from build123d import *

# Parameters (mm, degrees)
EXTRUDE1_DEPTH      = 228.73
CUT_EXTRUDE1_DEPTH  = 95
EXTRUDE2_DEPTH      = 50
EXTRUDE2_DEPTH_BACK = 100


with BuildPart() as part:
    # Sketch1 → Extrude1 (new body)
    with BuildSketch(Plane(origin=(0, 0, 0), x_dir=(1, 0, 0), z_dir=(0, 1, 0))):
        Polygon((0, 0), (91.923881554, 91.923881554), (0, 183.847763109), (-91.923881554, 91.923881554), align=None)
    extrude(amount=EXTRUDE1_DEPTH)

    # Sketch2 → Cut-Extrude1 (cut, symmetric)
    with BuildSketch(Plane(origin=(0, 0, 0), x_dir=(0, 0, -1), z_dir=(1, 0, 0))):
        Polygon((0, 100), (183.847763109, 228.731589612), (0, 228.731589612), align=None)
    extrude(amount=CUT_EXTRUDE1_DEPTH, both=True, mode=Mode.SUBTRACT)

    # Sketch3 → Extrude2 (add, two sides)
    with BuildSketch(Plane.XY) as extrude2_sk:
        with BuildLine():
            Line((-60, 0), (60, 0))
            add(Edge.make_bspline(
                [(-60, 0), (0, 300), (60, 0)],
                knots=[0, 0, 0, 1, 1, 1], degree=2))
        make_face()
    extrude(amount=EXTRUDE2_DEPTH)
    extrude(extrude2_sk.sketch, amount=-EXTRUDE2_DEPTH_BACK)


solid = part.part
Read the model definition and answer for the solid it produces. Units are mm, in the model's axes. A direction names the side the tool comes from. Give positions to 0.01 mm unless a question says otherwise; leave off trailing zeros. Write each loop counter-clockwise with the first axis right and the second up, starting at its lowest first coordinate (ties: lowest second). Pieces come first, ordered by that corner, then holes. Notation, with made-up numbers: M 75.5,15.25 L 79.5,15.25 A13 cw 79.5,19.25 Z; hole C 39.5,-10.5 d1. An arc over 180 degrees is marked long. One line per item, written item: value. Start each with the question number.
(1) Find section A-A (x = -74). Determine the outline of the cut face in (y, z), plus the area to 3 significant figures.
(2) Find section C-C (y = 181). Determine the outline of the cut face in (x, z).
(3) Find the intervals of material crossed by line 1 (Z direction, x = 73.5, y = 33); line 2 (X direction, y = 35.5, z = -163.5); line 3 (X direction, y = 65, z = -37), in increasing order.
(4) Flat-ended cylindrical pins translate along their axes: pin 1 Ø2 at (y, z) = (129.5, 15.5) entering from -X; pin 2 Ø10 at (x, y) = (51, 201.5) entering from +Z; pin 3 Ø12 at (y, z) = (104, 5.5) entering from +X; pin 4 Ø3 at (y, z) = (116.5, -69.5) entering from +X. Find the tip coordinate at first contact, or state that the pin passes through.
(5) A tool of negligible diameter and unlimited length cuts with its end or side. For faces 1 (the flat face through (1.3, 173.1, -104.4)), 2 (the flat face through (-67, 81, -67)), 3 (the flat face through (66, 81, -66)), from which of +Z, -Z, +X, -X, +Y, -Y can it reach the whole face along a straight path? Write none if from no direction.
(6) Find section B-B (z = -75.5). Determine the outline of the cut face in (x, y), plus the area to 3 significant figures.
Results below:
1. outline: M 0,-109.85 L 176.92,-109.85 L 151.82,-74 L 0,-74 Z
1. area: 5,890 mm^2
2. outline: M -68.17,-115.68 L 0,-183.85 L 68.17,-115.68 Z
3. line 1: z = -110.35 to -73.5
3. line 2: x = -20.35 to 20.35
3. line 3: x = -45.17 to 45.17
4. pin 1: stops at x = -22.72
4. pin 2: passes through
4. pin 3: stops at x = 35.33
4. pin 4: stops at x = 71
5. face 1: +Z, +Y
5. face 2: +Z, -X, +Y
5. face 3: +Z, +X, +Y
6. outline: M -75.5,0 L 75.5,0 L 75.5,152.87 L -75.5,152.87 Z
6. area: 23,100 mm^2
